The model under review builds one solid part; all positions refer to its coordinate system, in mm. Face numbers are marked on the shaded views. Give positions to 0.01 mm unless a question says otherwise; leave off trailing zeros. Write each loop counter-clockwise with the first axis right and the second up, starting at its lowest first coordinate (ties: lowest second). Pieces come first, ordered by that corner, then holes.
Autodesk Inventor part; units mm, degrees
ref_plane "YZ Plane" through (0, 0, 0) normal (1, 0, 0) x (0, 1, 0)
ref_plane "XZ Plane" through (0, 0, 0) normal (0, 1, 0) x (-1, 0, 0)
ref_plane "XY Plane" through (0, 0, 0) normal (0, 0, 1) x (1, 0, 0)
sketch "Sketch1" plane through (0, 0, 0) normal (0, 1, 0) x (-1, 0, 0)
  line L0 (40, 20) -> (-40, 20)
  line L1 (-40, 20) -> (-40, -20)
  line L2 (-40, -20) -> (40, -20)
  line L3 (40, -20) -> (40, 20)
  line L4 (40, 20) -> (-40, -20) construction
  line L5 (-40, 20) -> (40, -20) construction
  point P0 (0, 0)
  dimension "d0" = 80
  dimension "d1" = 40
extrude "Extrusion1" add sketch "Sketch1" along normal blind 3
sketch "Sketch2" plane through (0, 3, 0) normal (0, 1, 0) x (1, 0, 0)
  line L0 (-35, -12.5) -> (35, -12.5)
  line L1 (35, -12.5) -> (35, 12.5)
  line L2 (35, 12.5) -> (-35, 12.5)
  line L3 (-35, 12.5) -> (-35, -12.5)
  line L4 (-35, -12.5) -> (35, 12.5) construction
  line L5 (35, -12.5) -> (-35, 12.5) construction
  point P0 (0, 0)
  dimension "d4" = 70
  dimension "d5" = 25
extrude "Extrusion2" add sketch "Sketch2" along normal blind 10
sketch "Sketch3" plane through (0, 13, 0) normal (0, 1, 0) x (1, 0, 0)
  line L0 (33, 10.5) -> (-33, 10.5)
  line L1 (-33, 10.5) -> (-33, -10.5)
  line L2 (-33, -10.5) -> (33, -10.5)
  line L3 (33, -10.5) -> (33, 10.5)
  line L4 (33, 10.5) -> (-33, -10.5) construction
  line L5 (-33, 10.5) -> (33, -10.5) construction
  point P0 (0, 0)
  dimension "d8" = 66
  dimension "d9" = 21
extrude "Extrusion3" cut sketch "Sketch3" against normal blind 1.5
fillet "Fillet1" radius 1.5 4 edges at (0, 13, -10.5) (-33, 13, 0) (0, 13, 10.5) (33, 13, 0)
sketch "Sketch4" plane through (0, 3, 0) normal (0, 1, 0) x (1, 0, 0)
  line L0 (-40, 20) -> (-40, 16)
  line L1 (-40, 20) -> (-40, -20)
  line L2 (-40, 16) -> (-36, 16)
  circle A0 centre (-36, 16) radius 2
  line L3 (-40, 0) -> (40, 0)
  line L4 (40, -20) -> (40, 20)
  line L5 (40, 20) -> (-40, 20)
  line L6 (0, 20) -> (0, -20)
  line L7 (-40, -20) -> (40, -20)
  circle A1 centre (-36, -16) radius 2
  circle A2 centre (36, 16) radius 2
  circle A3 centre (36, -16) radius 2
  point P0 (0, 0)
  dimension "d13" = 4
  dimension "d14" = 4
  dimension "d15" = 4
extrude "Extrusion4" cut sketch "Sketch4" against normal blind 3 contours A0 | A1 | A2 | A3
properties part number "LCD"
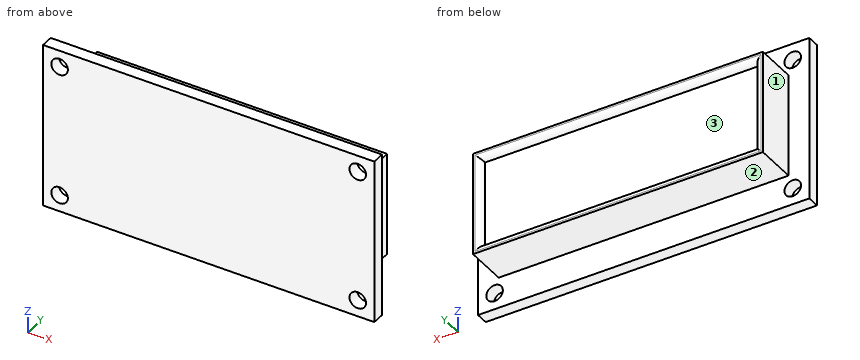
1) Insertion check: pin 1 (6.5 mm diameter, centred on x = 36, z = 16, fed in from +Y); pin 2 (3.5 mm diameter, centred on x = -36, z = 16, fed in from +Y); pin 3 (1.5 mm diameter, centred on x = 11, z = -12, fed in from -Y); pin 4 (3 mm diameter, centred on y = 9.5, z = 3, fed in from -X). Each pin has a flat end and moves straight along its axis. Give the tip position at first contact, or say it passes through.
2) The part is to be moulded in two halves that separate along X. For the marked faces 1, 2 and 3, say which applies: +X half, -X half, draft (parallel to the pull), parting line (faces both ways), or undercut.
3) Consider section B-B, the plane z = 16. Give the boundary of the cut face in (x, y), then the cut area to 3 significant figures.
4) To check wall thickness, follow probe 1 along Z at (x, y) = (36, 2.25); probe 2 along X at (y, z) = (1.8, 16); probe 3 along X at (y, z) = (5, -4). State the ranges of each line that lie inside material, in increasing order.
5) Consider section A-A, the plane x = -36. Give the boundary of the cut face in (y, z), then the cut area to 3 significant figures.
Answer block:
1. pin 1: stops at y = 3
1. pin 2: passes through
1. pin 3: stops at y = 0
1. pin 4: stops at x = -35
2. face 1: -X half
2. face 2: draft
2. face 3: undercut
3. outline: (-40, 0) - (-38, 0) - (-38, 3) - (-40, 3) - close; (-34, 0) - (34, 0) - (34, 3) - (-34, 3) - close; (38, 0) - (40, 0) - (40, 3) - (38, 3) - close
3. area: 216 mm2
4. probe 1: z = -20 to -18, -14 to 14, 18 to 20
4. probe 2: x = -40 to -38, -34 to 34, 38 to 40
4. probe 3: x = -35 to 35
5. outline: (0, -20) - (3, -20) - (3, -18) - (0, -18) - close; (0, -14) - (3, -14) - (3, 14) - (0, 14) - close; (0, 18) - (3, 18) - (3, 20) - (0, 20) - close
5. area: 96.0 mm2
